Source: CAD feature listing. Evaluate the final solid. Frame: model axes, mm. A direction names the side the tool comes from. Give positions to 0.01 mm unless a question says otherwise; leave off trailing zeros. Loops run counter-clockwise (first coordinate to the right, second up) from the corner with the lowest first, then second, coordinate; pieces in that order, holes last.
```python
from build123d import *

# Parameters (mm, degrees)
SKETCH2_W           = 150
SKETCH2_H           = 80
SKETCH2_R           = 1.5
BOSS_EXTRUDE1_DEPTH = 3
SKETCH3_R           = 5
SKETCH3_R_2         = 2.5
BOSS_EXTRUDE2_DEPTH = 50
SKETCH4_R           = 1.5
CUT_EXTRUDE1_DEPTH  = 10


with BuildPart() as part:
    # Sketch2 → Boss-Extrude1 (new body)
    with BuildSketch(Plane(origin=(0, 0, 0), x_dir=(1, 0, 0), z_dir=(0, 1, 0))):
        with Locations((-8.46473029, 1.825726141)):
            Rectangle(SKETCH2_W, SKETCH2_H)
        with Locations((-68.46473029, 11.325726141)):
            Circle(SKETCH2_R, mode=Mode.SUBTRACT)
        with Locations((-68.46473029, -7.674273859)):
            Circle(SKETCH2_R, mode=Mode.SUBTRACT)
        with Locations((-76.46473029, 11.325726141)):
            Circle(SKETCH2_R, mode=Mode.SUBTRACT)
        with Locations((-76.46473029, -7.674273859)):
            Circle(SKETCH2_R, mode=Mode.SUBTRACT)
        with Locations((51.53526971, -7.674273859)):
            Circle(SKETCH2_R, mode=Mode.SUBTRACT)
        with Locations((59.53526971, -7.674273859)):
            Circle(SKETCH2_R, mode=Mode.SUBTRACT)
        with Locations((59.53526971, 11.325726141)):
            Circle(SKETCH2_R, mode=Mode.SUBTRACT)
        with Locations((51.53526971, 11.325726141)):
            Circle(SKETCH2_R, mode=Mode.SUBTRACT)
    extrude(amount=-BOSS_EXTRUDE1_DEPTH)

    # Sketch3 → Boss-Extrude2 (add)
    with BuildSketch(Plane(origin=(0, 0, 0), x_dir=(1, 0, 0), z_dir=(0, 1, 0))):
        with Locations((-73.46473029, 31.825726141)):
            Circle(SKETCH3_R)
        with Locations((-73.46473029, 31.825726141)):
            Circle(SKETCH3_R_2, mode=Mode.SUBTRACT)
        with Locations((56.53526971, 31.825726141)):
            Circle(SKETCH3_R)
        with Locations((56.53526971, 31.825726141)):
            Circle(SKETCH3_R_2, mode=Mode.SUBTRACT)
        with Locations((56.53526971, -28.174273859)):
            Circle(SKETCH3_R)
        with Locations((56.53526971, -28.174273859)):
            Circle(SKETCH3_R_2, mode=Mode.SUBTRACT)
        with Locations((-73.46473029, -28.174273859)):
            Circle(SKETCH3_R)
        with Locations((-73.46473029, -28.174273859)):
            Circle(SKETCH3_R_2, mode=Mode.SUBTRACT)
    extrude(amount=BOSS_EXTRUDE2_DEPTH)

    # Sketch4 → Cut-Extrude1 (cut)
    with BuildSketch(Plane.XZ.offset(3)):
        with Locations((-26.96473029, 16.674273859)):
            Circle(SKETCH4_R)
        with Locations((10.03526971, 16.674273859)):
            Circle(SKETCH4_R)
        with Locations((10.03526971, -20.325726141)):
            Circle(SKETCH4_R)
        with Locations((-26.353154243, -20.325726141)):
            Circle(SKETCH4_R)
    extrude(amount=-CUT_EXTRUDE1_DEPTH, mode=Mode.SUBTRACT)


solid = part.part
```
(1) Reachability of faces 5 (the cylindrical face through (54.551, 24.65, -30.305)), 6 (the cylindrical face through (-77.963, -1.479, -11.392)) from +Z, -Z, +X, -X, +Y, -Y: full face, straight path, thin tool, end or side. Return the list, or none.
A:
face 5: +Y
face 6: +Y, -Y
(2) Section C-C, the plane z = 0. Return the cut outline in (x, y), then the cut area to 3 significant figures.
A:
outline: (-83.46, -3) - (66.54, -3) - (66.54, 0) - (-83.46, 0) - close
area: 450 mm2
(3) Section B-B, the plane x = -4. Return the cut outline in (y, z), then the cut area to 3 significant figures.
A:
outline: (-3, -41.83) - (0, -41.83) - (0, 38.17) - (-3, 38.17) - close
area: 240 mm2
(4) Ray query, line 1 along X through (y, z) = (1, -33.5); line 2 along Y through (x, z) = (33, -2.5); line 3 along X through (y, z) = (11.5, 29.5). Return the intervals inside material, ascending.
A:
line 1: x = -78.18 to -75.32, -71.61 to -68.75, 51.82 to 54.68, 58.39 to 61.25
line 2: y = -3 to 0
line 3: x = -78.29 to -75.58, -71.35 to -68.64, 51.71 to 54.42, 58.65 to 61.36
(5) Mould query, pull axis X, two halves, no side actions, for faces 1 (the cylindrical face through (52.85, 24.65, 24.795)), 2 (the flat face through (66.535, -1, -1)), 3 (the cylindrical face through (-78.46, 24.65, -32.05)), 4 (the flat face through (-76, 50, -31)). Classes: pulls with the +X half, pulls with the -X half, needs draft (parallel to the pull), parting line crosses it, or undercut.
A:
face 1: undercut
face 2: pulls with the +X half
face 3: undercut
face 4: needs draft
(6) Section A-A, the plane y = 9. Return the cut outline in (x, z), then the cut area to 3 significant figures.
A:
outline: circle Ø10 at (-73.46, -31.83); circle Ø10 at (-73.46, 28.17); circle Ø10 at (56.54, -31.83); circle Ø10 at (56.54, 28.17); hole circle Ø5 at (-73.46, -31.83); hole circle Ø5 at (-73.46, 28.17); hole circle Ø5 at (56.54, -31.83); hole circle Ø5 at (56.54, 28.17)
area: 236 mm2
(7) First-contact query: pin 1 (6 mm diameter, centred on x = -63.5, z = -8.5, fed in from +Y); pin 2 (1.8 mm diameter, centred on x = 51.54, z = -11.33, fed in from -Y); pin 3 (4 mm diameter, centred on x = -68, y = 14, fed in from +Z). Flat tips, straight axial feed; report the tip coordinate or a pass-through.
A:
pin 1: stops at y = 0
pin 2: passes through
pin 3: stops at z = 31.78
